from build123d import *

# Parameters (mm, degrees)
SKETCH1_R           = 18
SKETCH1_R_2         = 8
BOSS_EXTRUDE1_DEPTH = 8
SKETCH2_R           = 8
SKETCH2_R_2         = 6
BOSS_EXTRUDE2_DEPTH = 1.6
SKETCH3_W           = 40
SKETCH3_H           = 20
CUT_EXTRUDE1_DEPTH  = 9
CUT_EXTRUDE2_REACH  = 19
SKETCH5_R           = 1.6
CUT_EXTRUDE3_REACH  = 27
CUT_EXTRUDE3_START  = -8


with BuildPart() as part:
    # Sketch1 → Boss-Extrude1 (new body)
    with BuildSketch(Plane(origin=(0, 0, 0), x_dir=(1, 0, 0), z_dir=(0, 1, 0))):
        Circle(SKETCH1_R)
        Circle(SKETCH1_R_2, mode=Mode.SUBTRACT)
    extrude(amount=BOSS_EXTRUDE1_DEPTH)

    # Sketch2 → Boss-Extrude2 (add)
    with BuildSketch(Plane(origin=(0, 0, 0), x_dir=(1, 0, 0), z_dir=(0, 1, 0))):
        Circle(SKETCH2_R)
        Circle(SKETCH2_R_2, mode=Mode.SUBTRACT)
    extrude(amount=BOSS_EXTRUDE2_DEPTH)

    # Sketch3 → Cut-Extrude1 (cut, through all)
    with BuildSketch(Plane(origin=(0, 8, 0), x_dir=(1, 0, 0), z_dir=(0, 1, 0))):
        with Locations((0, -9)):
            Rectangle(SKETCH3_W, SKETCH3_H)
    extrude(amount=-CUT_EXTRUDE1_DEPTH, mode=Mode.SUBTRACT)

    # Sketch5 → Cut-Extrude2 (cut, up to next)
    with BuildSketch(Plane.XY.offset(-1), mode=Mode.PRIVATE) as cut_extrude2_sk1:
        with Locations((-12.954727344, 4)):
            Circle(SKETCH5_R)
    cut_extrude2_tool1 = extrude(cut_extrude2_sk1.sketch, amount=-CUT_EXTRUDE2_REACH, mode=Mode.PRIVATE) & part.part
    add(cut_extrude2_tool1.solids().sort_by_distance((-12.954727, 4, -1))[0], mode=Mode.SUBTRACT)
    # Sketch5 → Cut-Extrude2 (cut, up to next)
    with BuildSketch(Plane.XY.offset(-1), mode=Mode.PRIVATE) as cut_extrude2_sk2:
        with Locations((12.954727344, 4)):
            Circle(SKETCH5_R)
    cut_extrude2_tool2 = extrude(cut_extrude2_sk2.sketch, amount=-CUT_EXTRUDE2_REACH, mode=Mode.PRIVATE) & part.part
    add(cut_extrude2_tool2.solids().sort_by_distance((12.954727, 4, -1))[0], mode=Mode.SUBTRACT)

    # Sketch6 → Cut-Extrude3 (cut, up to next)
    with BuildSketch(Plane.XY.offset(-1).offset(CUT_EXTRUDE3_START), mode=Mode.PRIVATE) as cut_extrude3_sk1:
        Polygon((-9.721565837, 4), (-11.338146591, 6.8), (-14.571308098, 6.8), (-16.187888852, 4), (-14.571308098, 1.2), (-11.338146591, 1.2), align=None)
    cut_extrude3_tool1 = extrude(cut_extrude3_sk1.sketch, amount=-CUT_EXTRUDE3_REACH, mode=Mode.PRIVATE) & part.part
    add(cut_extrude3_tool1.solids().sort_by_distance((-12.954727, 4, -9))[0], mode=Mode.SUBTRACT)
    # Sketch6 → Cut-Extrude3 (cut, up to next)
    with BuildSketch(Plane.XY.offset(-1).offset(CUT_EXTRUDE3_START), mode=Mode.PRIVATE) as cut_extrude3_sk2:
        Polygon((16.187888852, 4), (14.571308098, 6.8), (11.338146591, 6.8), (9.721565837, 4), (11.338146591, 1.2), (14.571308098, 1.2), align=None)
    cut_extrude3_tool2 = extrude(cut_extrude3_sk2.sketch, amount=-CUT_EXTRUDE3_REACH, mode=Mode.PRIVATE) & part.part
    add(cut_extrude3_tool2.solids().sort_by_distance((12.954727, 4, -9))[0], mode=Mode.SUBTRACT)


solid = part.part
Can you work these out from the model? Positions are in its coordinate system, mm. A direction names the side the tool comes from. Round coordinates to 2 decimals unless told otherwise and drop trailing zeros. Loops run counter-clockwise (first coordinate to the right, second up) from the corner with the lowest first, then second, coordinate; pieces in that order, holes last. Notation, with made-up numbers: (-10.75, 70.25) - (3.25, 70.25) arc R9 ccw to (3.25, 77.25) - close; hole circle Ø3 at (67, -34). An arc over 180 degrees is marked (long way). Write item = value, one per line. Start each with the question number.
(1) If we section it at B-B (z = -12.5): Please give me the cut outline in (x, y), and give its area (3 significant figures).
(2) For faces 1 (the face through (0, 4, -18)), 2 (the face through (-0.6, 1.6, -6.3)), 3 (the face through (13, 1.2, -11)), which set-ups out of +Z, -Z, +X, -X, +Y, -Y let a thin tool reach every point of the face, with its end or its side?
(3) For P1, Ø1, axis at y = 6, z = -15.5, coming from the +X side, with a flat end and sliding along its axis, tell me the tip position at first contact or that it passes through.
(4) If I drill on probe 1 along X at (y, z) = (3.25, -4); probe 2 along Z at (x, y) = (12, 6.75); probe 3 along Y at (x, z) = (-11.5, -2.75), over which ranges is the centre line in solid material (lowest first)? Write a range as [from, to].
(5) If we section it at D-D (x = -9): Please give me the cut outline in (y, z), and give its area (3 significant figures).
(6) If we section it at C-C (y = 0.5): Please give me the cut outline in (x, z), and give its area (3 significant figures).
(7) If we mould it in two halves opening along Y, with no side actions, what happens to faces 4 (the face through (0, 8, -10)), 5 (the face through (-14.96, 6.13, -9.6)), 6 (the face through (0, 5, -8))? For each: released by +Y, released by -Y, zero draft, split by the parting line, or undercut.
(8) If we section it at A-A (x = -13.5): Please give me the cut outline in (y, z), and give its area (3 significant figures).
Ans:
q1.outline = (-12.95, 0) - (12.95, 0) - (12.95, 1.2) - (11.34, 1.2) - (9.72, 4) - (11.34, 6.8) - (12.95, 6.8) - (12.95, 8) - (-12.95, 8) - (-12.95, 6.8) - (-11.34, 6.8) - (-9.72, 4) - (-11.34, 1.2) - (-12.95, 1.2) - close
q1.area = 180 mm²
q2.face_1 = -Z, +Y, -Y
q2.face_2 = +Z, +Y
q2.face_3 = -Z
q3.P1 = 9.95
q4.probe_1 = [-17.55, -14.37], [-11.54, -6.93], [6.93, 11.54], [14.37, 17.55]
q4.probe_2 = [-9, -1]
q4.probe_3 = [0, 3.33], [4.67, 8]
q5.outline = (0, -15.59) - (8, -15.59) - (8, -1) - (0, -1) - close
q5.area = 117 mm²
q6.outline = (-17.97, -1) arc R18 ccw to (17.97, -1) - (5.92, -1) arc R6 cw to (-5.92, -1) - close
q6.area = 428 mm²
q7.face_4 = released by +Y
q7.face_5 = undercut
q7.face_6 = zero draft
q8.outline = (0, -11.91) - (1.2, -11.91) - (1.2, -9) - (2.5, -9) - (2.5, -1) - (0, -1) - close; (5.5, -9) - (6.8, -9) - (6.8, -11.91) - (8, -11.91) - (8, -1) - (5.5, -1) - close
q8.area = 46.9 mm²
